Autodesk Inventor part; units mm, degrees
ref_plane "YZ Plane" through (0, 0, 0) normal (1, 0, 0) x (0, 1, 0)
ref_plane "XZ Plane" through (0, 0, 0) normal (0, 1, 0) x (-1, 0, 0)
ref_plane "XY Plane" through (0, 0, 0) normal (0, 0, 1) x (1, 0, 0)
sketch "Эскиз1" plane through (0, 0, 0) normal (0, 1, 0) x (-1, 0, 0)
  circle A0 centre (0, 0) radius 2.5
  circle A1 centre (0, 0) radius 10
  dimension "d0" = 5
  dimension "d1" = 20
extrude "Выдавливание1" add sketch "Эскиз1" along normal blind 22
sketch "Эскиз2" plane through (0, 22, 0) normal (0, 1, 0) x (1, 0, 0)
  circle A0 centre (0, 0) radius 10
extrude "Выдавливание2" add sketch "Эскиз2" along normal blind 485
thread "Резьба1"
chamfer "Фаска1" distance 2 angle 45 1 edges at (-10, 507, 0)
sketch "Эскиз3" plane through (0, 507, 0) normal (0, 1, 0) x (1, 0, 0)
  circle A0 centre (0, 0) radius 2.5
  circle A1 centre (0, 0) radius 15
  dimension "d11" = 30
extrude "Выдавливание3" add sketch "Эскиз3" against normal blind 5
properties part number "Резьбовой винт"
CAD build for the part. Positions are in the model's coordinates, mm. A direction names the side the tool comes from. Round coordinates to 2 decimals unless told otherwise and drop trailing zeros. Loops run counter-clockwise (first coordinate to the right, second up) from the corner with the lowest first, then second, coordinate; pieces in that order, holes last. Notation, with made-up numbers: M 49.25,-18.75 L 103.25,-18.75 A29 cw 103.25,15.25 Z; hole C 76,65.5 d5. An arc over 180 degrees is marked long. Return JSON: item names as keys, results as strings. Group by question number.
(1) Wall check: probe 1 along Z at (x, y) = (0, 14.5); probe 2 along Y at (x, z) = (-10, 6.5); probe 3 along Y at (x, z) = (0.5, -1.25). Give the ranges that are in metal, low to high. Write a range as [from, to].
(2) Saw through at A-A, the plane y = 324.5. List the corners of the cut face in (x, z), and give its area (3 significant figures).
(3) Tool access for faces 1 (the flat face through (3, 502, 10)), 2 (the flat face through (-2, 0, -2)): list every direction of +Z, -Z, +X, -X, +Y, -Y with a clear straight run to the whole face (end or side of a thin tool).
(4) Drop flat-ended pins along their axis: P1, Ø5, axis at x = 9, y = 120, coming from the -Z side; P2, Ø1.5, axis at x = 0, z = 0, coming from the -Y side; P3, Ø1.5, axis at y = 210, z = -2, coming from the +X side. Give the stop position or say it passes through.
Answer list:
{
 "1": {"probe 1": "[-10, -2.5], [2.5, 10]", "probe 2": "[502, 507]", "probe 3": "[22, 507]"},
 "2": {"outline": "C 0,0 d20", "area": "314 mm2"},
 "3": {"face 1": "-Y", "face 2": "+Z, -Z, +X, -X, -Y"},
 "4": {"P1": "z = -7.6", "P2": "y = 22", "P3": "x = 9.92"}
}
